Check sheet for the drawn part. Datum: minimum x, y, z corner. Units: mm. Give positions to 0.01 mm unless a question says otherwise; leave off trailing zeros. Loops run counter-clockwise (first coordinate to the right, second up) from the corner with the lowest first, then second, coordinate; pieces in that order, holes last.
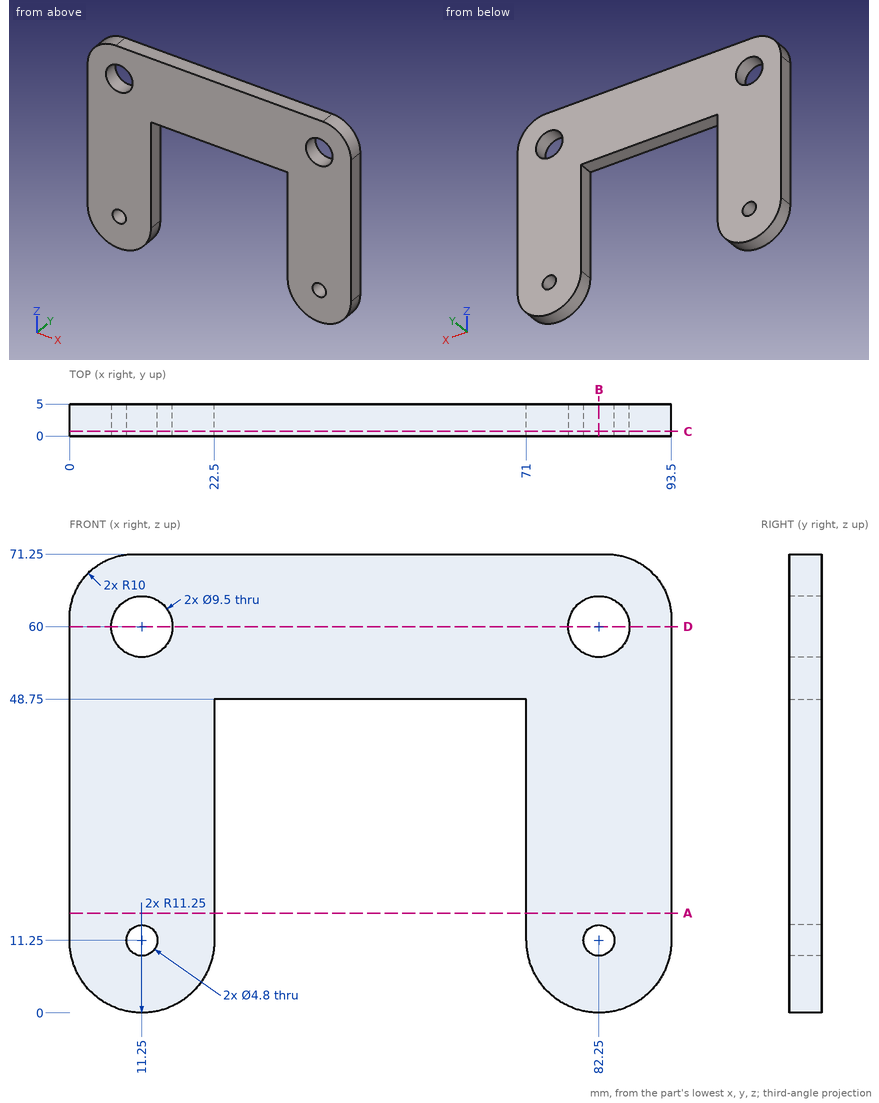
(1) Gauge pin test, flat ends, axial feed: pin 1 Ø1.5 at (y, z) = (1.5, 23) entering from -X; pin 2 Ø2.5 at (x, y) = (57.5, 1.5) entering from -Z. Record the tip position at first contact, or that the pin passes through.
(2) Section check C-C on y = 0.75. Record the boundary of the cut face in (x, z), plus the area to 3 significant figures.
(3) Section check D-D on z = 60. Record the boundary of the cut face in (x, y), plus the area to 4 significant figures.
(4) Section check B-B on x = 82.25. Record the boundary of the cut face in (y, z), plus the area to 3 significant figures.
(5) Material ranges on line 1 (Z direction, x = 82.25, y = 2.9); line 2 (X direction, y = 3.45, z = 11.25); line 3 (X direction, y = 3.6, z = 60), recorded low to high.
(6) Section check A-A on z = 15.5. Record the boundary of the cut face in (x, y), plus the area to 3 significant figures.
Computed values:
1. pin 1: stops at x = 0
1. pin 2: stops at z = 48.75
2. outline: (0, 11.25) arc R11.25 ccw to (22.5, 11.25) - (22.5, 48.75) - (71, 48.75) - (71, 11.25) arc R11.25 ccw to (93.5, 11.25) - (93.5, 61.25) arc R10 ccw to (83.5, 71.25) - (10, 71.25) arc R10 ccw to (0, 61.25) - close; hole circle Ø9.5 at (11.25, 60); hole circle Ø4.8 at (11.25, 11.25); hole circle Ø9.5 at (82.25, 60); hole circle Ø4.8 at (82.25, 11.25)
2. area: 3,970 mm2
3. outline: (0, 0) - (6.5, 0) - (6.5, 5) - (0, 5) - close; (16, 0) - (77.5, 0) - (77.5, 5) - (16, 5) - close; (87, 0) - (93.5, 0) - (93.5, 5) - (87, 5) - close
3. area: 372.5 mm2
4. outline: (0, 0) - (5, 0) - (5, 8.85) - (0, 8.85) - close; (0, 13.65) - (5, 13.65) - (5, 55.25) - (0, 55.25) - close; (0, 64.75) - (5, 64.75) - (5, 71.25) - (0, 71.25) - close
4. area: 285 mm2
5. line 1: z = 0 to 8.85, 13.65 to 55.25, 64.75 to 71.25
5. line 2: x = 0 to 8.85, 13.65 to 22.5, 71 to 79.85, 84.65 to 93.5
5. line 3: x = 0 to 6.5, 16 to 77.5, 87 to 93.5
6. outline: (0, 0) - (22.5, 0) - (22.5, 5) - (0, 5) - close; (71, 0) - (93.5, 0) - (93.5, 5) - (71, 5) - close
6. area: 225 mm2
